Here's the drawing with two shaded views (mm, measured from the low corner). I have some questions. A direction names the side the tool comes from. Coordinates: 2 decimals unless noted, no trailing zeros. Write each loop counter-clockwise with the first axis right and the second up, starting at its lowest first coordinate (ties: lowest second). Pieces come first, ordered by that corner, then holes.
Item 1: If we section it at D-D (y = 18.75): Count the separate pieces of the cut face and the enclosed holes in it, then the cut area to 3 significant figures.
Item 2: If we section it at C-C (z = 15.5): Please give me the cut outline in (x, y), then the cut area to 3 significant figures.
Item 3: For the marked faces 1, 2, 3, 4 and 5, which set-ups out of +Z, -Z, +X, -X, +Y, -Y let a thin tool reach every point of the face, with its end or its side?
Item 4: If we section it at B-B (x = 96.5): Please give me the cut outline in (y, z).
Item 5: If we section it at A-A (z = 6.35): Please give me the cut outline in (x, y).
Item 6: If I drill on line 1 (X direction, y = 19, z = 32) (1 decimal); line 2 (X direction, y = 18, z = 48); line 3 (Z direction, x = 113.03, y = 6.5), over which ranges is the centre line in solid material (lowest first)?
Item 7: I'm going to push flat-ended pins straight in: pin 1 Ø10 at (x, z) = (59, 32) entering from +Y; pin 2 Ø6.5 at (y, z) = (1.5, 32.5) entering from -X; pin 3 Ø10 at (x, y) = (21, 5) entering from +Z; pin 4 Ø4 at (x, y) = (12.5, 7.5) entering from -Z. Where does each tip first touch, or does it pass through?
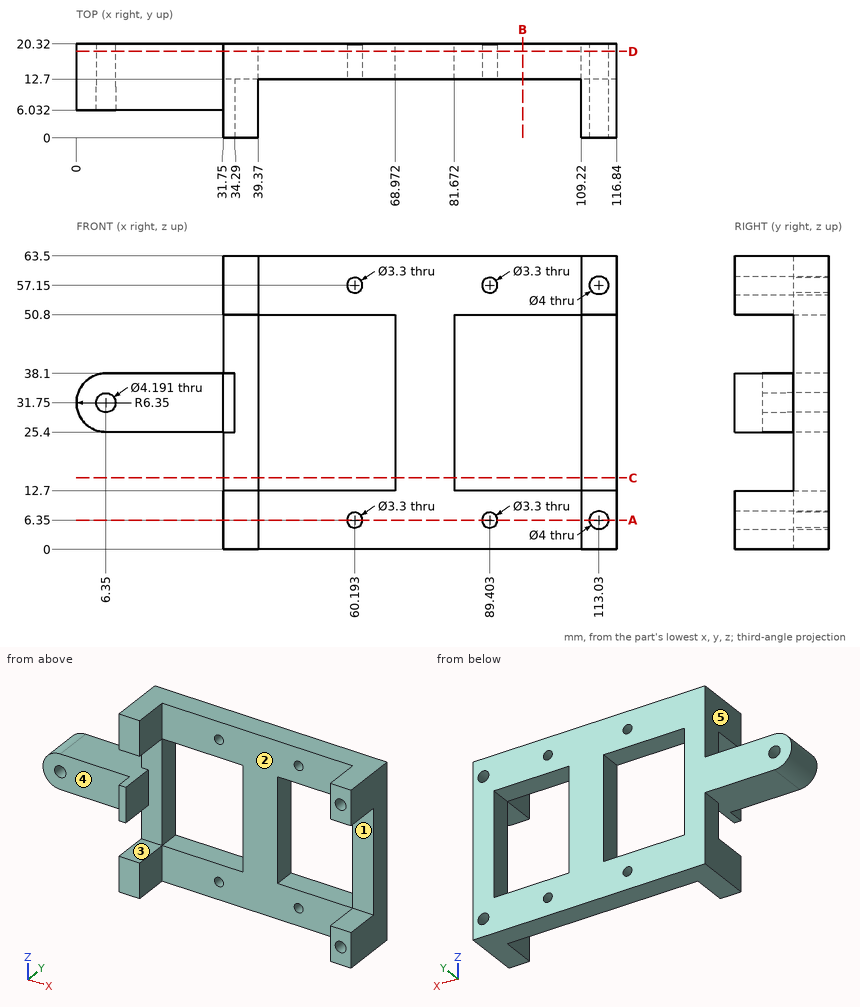
Answer list:
1. separate pieces: 1
1. enclosed holes: 9
1. area: 3,540 mm2
2. outline: (31.75, 12.7) - (39.37, 12.7) - (39.37, 20.32) - (31.75, 20.32) - close; (68.97, 12.7) - (81.67, 12.7) - (81.67, 20.32) - (68.97, 20.32) - close; (109.22, 12.7) - (116.84, 12.7) - (116.84, 20.32) - (109.22, 20.32) - close
2. area: 213 mm2
3. face 1: +X, -Y
3. face 2: +Z, -Z, -Y
3. face 3: +X, -X, -Y
3. face 4: +Z, -Z, -X, -Y
3. face 5: +Z, -X, +Y, -Y
4. outline: (12.7, 0) - (20.32, 0) - (20.32, 12.7) - (12.7, 12.7) - close; (12.7, 50.8) - (20.32, 50.8) - (20.32, 63.5) - (12.7, 63.5) - close
5. outline: (31.75, 0) - (39.37, 0) - (39.37, 12.7) - (58.54, 12.7) - (58.54, 20.32) - (31.75, 20.32) - close; (61.84, 12.7) - (87.75, 12.7) - (87.75, 20.32) - (61.84, 20.32) - close; (91.05, 12.7) - (109.22, 12.7) - (109.22, 0) - (111.03, 0) - (111.03, 20.32) - (91.05, 20.32) - close; (115.03, 0) - (116.84, 0) - (116.84, 20.32) - (115.03, 20.32) - close
6. line 1: x = 0 to 4.3, 8.4 to 39.4, 69 to 81.7, 109.2 to 116.8
6. line 2: x = 31.75 to 39.37, 68.97 to 81.67, 109.22 to 116.84
6. line 3: z = 0 to 4.35, 8.35 to 12.7, 50.8 to 55.15, 59.15 to 63.5
7. pin 1: passes through
7. pin 2: stops at x = 31.75
7. pin 3: stops at z = 38.1
7. pin 4: stops at z = 25.4
